Work out the finished part from the listing and answer in its coordinate system (mm). A direction names the side the tool comes from. Give positions to 0.01 mm unless a question says otherwise; leave off trailing zeros. Loops run counter-clockwise (first coordinate to the right, second up) from the corner with the lowest first, then second, coordinate; pieces in that order, holes last. Notation, with made-up numbers: (85.5, -26.5) - (109.5, -26.5) arc R20 ccw to (109.5, -9.5) - close; hole circle Ø1 at (1.25, 71.25). An arc over 180 degrees is marked (long way). One line per question, with ' | ' between items.
from build123d import *

# Parameters (mm, degrees)
SKETCH_1_R                                     = 31
FOOT_125X100_R10_T8_OPEN_D62_DEPTH             = 8
SKETCH_2_R                                     = 3.3
M6_GRID25_100X75_DEPTH                         = 8
SKETCH_3_R                                     = 34
SKETCH_3_R_2                                   = 31
HOLLOW_COLUMN_OD68_ID62_TOZ134_DEPTH           = 126
SKETCH_5_R                                     = 34
SKETCH_5_R_2                                   = 30.6
BOTTOM_CAP_WRAP_OD68_ID61P2_H6_DEPTH           = 6
STRAIGHT_TRIANGULAR_RIB_T4_NO_FILLETS_X_DEPTH  = 4
STRAIGHT_TRIANGULAR_RIB_T4_NO_FILLETS_Y_DEPTH  = 4
SKETCH_8_R                                     = 1.7
STATOR_4XM3_PCD25_THROUGH_WEB_DEPTH            = 6
SKETCH_9_R                                     = 3.3
UNDERSIDE_BOLT_AND_DRIVER_WELLS_D6P6_DEPTH     = 24
INNER_WALL_WIRE_GROOVE_W14_R2_DEPTH40_NO_DEPTH = 40
BOTTOM_REAR_OFFSET_WIRE_EXIT_14X10_45DEG_DEPTH = 25


with BuildPart() as part:
    # 草图1 → Foot_125x100_R10_T8_open_D62 (new body)
    with BuildSketch(Plane.XY):
        with BuildLine():
            Line((-52.5, -50), (52.5, -50))
            ThreePointArc((52.5, -50), (59.571067812, -47.071067812), (62.5, -40))
            Line((62.5, -40), (62.5, 40))
            ThreePointArc((62.5, 40), (59.571067812, 47.071067812), (52.5, 50))
            Line((52.5, 50), (-52.5, 50))
            ThreePointArc((-52.5, 50), (-59.571067812, 47.071067812), (-62.5, 40))
            Line((-62.5, 40), (-62.5, -40))
            ThreePointArc((-62.5, -40), (-59.571067812, -47.071067812), (-52.5, -50))
        make_face()
        Circle(SKETCH_1_R, mode=Mode.SUBTRACT)
    extrude(amount=FOOT_125X100_R10_T8_OPEN_D62_DEPTH)

    # 草图2 → M6_grid25_100x75 (cut)
    with BuildSketch(Plane.XY.offset(8)):
        with Locations((-50, -37.5)):
            Circle(SKETCH_2_R)
        with Locations((-50, 37.5)):
            Circle(SKETCH_2_R)
        with Locations((50, -37.5)):
            Circle(SKETCH_2_R)
        with Locations((50, 37.5)):
            Circle(SKETCH_2_R)
    extrude(amount=-M6_GRID25_100X75_DEPTH, mode=Mode.SUBTRACT)

    # 草图3 → Hollow_column_OD68_ID62_toZ134 (add)
    with BuildSketch(Plane.XY.offset(8)):
        Circle(SKETCH_3_R)
        Circle(SKETCH_3_R_2, mode=Mode.SUBTRACT)
    extrude(amount=HOLLOW_COLUMN_OD68_ID62_TOZ134_DEPTH)

    # 草图4 → Integral_motor_seat_45deg_internal_closure (revolve)
    with BuildSketch(Plane(origin=(0, 0, 0), x_dir=(1, 0, 0), z_dir=(0, 1, 0)), mode=Mode.PRIVATE) as integral_motor_seat_45deg_internal_closu_sk:
        Polygon((7, -131), (31, -107), (34, -107), (34, -134), (7, -134), align=None)
    revolve(integral_motor_seat_45deg_internal_closu_sk.sketch.rotate(Axis((0, 0, 0), (0, 0, 1)), 180), axis=Axis((0, 0, 0), (0, 0, 1)))

    # 草图5 → Bottom_cap_wrap_OD68_ID61p2_H6 (add)
    with BuildSketch(Plane.XY.offset(134)):
        Circle(SKETCH_5_R)
        Circle(SKETCH_5_R_2, mode=Mode.SUBTRACT)
    extrude(amount=BOTTOM_CAP_WRAP_OD68_ID61P2_H6_DEPTH)

    # 草图6 → Straight_triangular_rib_T4_no_fillets_x (add)
    with BuildSketch(Plane(origin=(-2, 0, 0), x_dir=(0, 0, -1), z_dir=(1, 0, 0))):
        Polygon((-8, -32), (-8, -46), (-22, -32), align=None)
        Polygon((-8, 32), (-8, 46), (-22, 32), align=None)
    extrude(amount=STRAIGHT_TRIANGULAR_RIB_T4_NO_FILLETS_X_DEPTH)

    # 草图7 → Straight_triangular_rib_T4_no_fillets_y (add)
    with BuildSketch(Plane(origin=(0, -2, 0), x_dir=(1, 0, 0), z_dir=(0, 1, 0))):
        Polygon((-32, -8), (-56, -8), (-32, -32), align=None)
        Polygon((32, -8), (56, -8), (32, -32), align=None)
    extrude(amount=STRAIGHT_TRIANGULAR_RIB_T4_NO_FILLETS_Y_DEPTH)

    # 草图8 → Stator_4xM3_PCD25_through_web (cut)
    with BuildSketch(Plane.XY.offset(134)):
        with Locations((12.5, 0)):
            Circle(SKETCH_8_R)
        with Locations((0, 12.5)):
            Circle(SKETCH_8_R)
        with Locations((-12.5, 0)):
            Circle(SKETCH_8_R)
        with Locations((0, -12.5)):
            Circle(SKETCH_8_R)
    extrude(amount=-STATOR_4XM3_PCD25_THROUGH_WEB_DEPTH, mode=Mode.SUBTRACT)

    # 草图9 → Underside_bolt_and_driver_wells_D6p6 (cut)
    with BuildSketch(Plane.XY.offset(128)):
        with Locations((12.5, 0)):
            Circle(SKETCH_9_R)
        with Locations((0, 12.5)):
            Circle(SKETCH_9_R)
        with Locations((-12.5, 0)):
            Circle(SKETCH_9_R)
        with Locations((0, -12.5)):
            Circle(SKETCH_9_R)
    extrude(amount=-UNDERSIDE_BOLT_AND_DRIVER_WELLS_D6P6_DEPTH, mode=Mode.SUBTRACT)

    # 草图10 → Inner_wall_wire_groove_W14_R2_depth40_no_external_bulge (cut)
    with BuildSketch(Plane.XY.offset(134)):
        with BuildLine():
            Line((-5, 19.5), (5, 19.5))
            ThreePointArc((5, 19.5), (6.414213562, 20.085786438), (7, 21.5))
            Line((7, 21.5), (7, 29.5))
            ThreePointArc((7, 29.5), (6.414213562, 30.914213562), (5, 31.5))
            Line((5, 31.5), (-5, 31.5))
            ThreePointArc((-5, 31.5), (-6.414213562, 30.914213562), (-7, 29.5))
            Line((-7, 29.5), (-7, 21.5))
            ThreePointArc((-7, 21.5), (-6.414213562, 20.085786438), (-5, 19.5))
        make_face()
    extrude(amount=-INNER_WALL_WIRE_GROOVE_W14_R2_DEPTH40_NO_DEPTH, mode=Mode.SUBTRACT)

    # 草图11 → Bottom_rear_offset_wire_exit_14x10_45deg_roof (cut)
    with BuildSketch(Plane(origin=(0, 40, 0), x_dir=(1, 0, 0), z_dir=(0, 1, 0))):
        Polygon((9, -8), (23, -8), (23, -18), (16, -25), (9, -18), align=None)
    extrude(amount=-BOTTOM_REAR_OFFSET_WIRE_EXIT_14X10_45DEG_DEPTH, mode=Mode.SUBTRACT)


solid = part.part
1. Find section D-D on z = 39. Write down the section's boundary in (x, y).
Evaluation:
outline: circle Ø68 at (0, 0); hole circle Ø62 at (0, 0)
2. Consider L1, parallel to Y at x = 0, z = 135; L2, parallel to Y at x = 0, z = 126; L3, parallel to Y at x = -9.5, z = 125. Determine where each line is inside the solid, lowest interval first.
Evaluation:
L1: -34 to -30.6, 30.6 to 34 | L2: -34 to -15.8, 15.8 to 19.5, 31.5 to 34 | L3: -32.65 to -8.87, 8.87 to 32.65
3. Which of the six approach directions +Z, -Z, +X, -X, +Y, -Y give full straight-line access (tool end or side, diameter ignored) to faces 4 (the flat face through (40, 2, 14)), 5 (the flat face through (2, -39, 13)), 6 (the flat face through (13, 30, 22)), 7 (the cylindrical face through (-6.633, -29.872, 136.958)), 8 (the flat face through (-14.2, 0.8, 128))?
Evaluation:
face 4: +Z, +X, +Y | face 5: +Z, +X, -Y | face 6: +Y | face 7: +Z | face 8: -Z
4. Find section B-B on y = 37.5. Write down the section's boundary in (x, z), then the cut area to 3 significant figures.
Evaluation:
outline: (-62.5, 0) - (-53.3, 0) - (-53.3, 8) - (-62.5, 8) - close; (-46.7, 0) - (46.7, 0) - (46.7, 8) - (2, 8) - (2, 16.5) - (-2, 16.5) - (-2, 8) - (-46.7, 8) - close; (53.3, 0) - (62.5, 0) - (62.5, 8) - (53.3, 8) - close | area: 928 mm2
5. Find section C-C on z = 103. Write down the section's boundary in (x, y), then the cut area to 3 significant figures.
Evaluation:
outline: circle Ø68 at (0, 0); hole (-6.86, 30.23) arc R31 ccw (long way) to (6.86, 30.23) arc R2 ccw to (5, 31.5) - (-5, 31.5) arc R2 ccw to start | area: 604 mm2
6. Find section A-A on x = 50. Write down the section's boundary in (y, z), then the cut area to 3 significant figures.
Evaluation:
outline: (-50, 0) - (-40.8, 0) - (-40.8, 8) - (-50, 8) - close; (-34.2, 0) - (34.2, 0) - (34.2, 8) - (2, 8) - (2, 14) - (-2, 14) - (-2, 8) - (-34.2, 8) - close; (40.8, 0) - (50, 0) - (50, 8) - (40.8, 8) - close | area: 718 mm2
7. Flat-ended cylindrical pins translate along their axes: pin 1 (4 mm diameter, centred on x = 12.5, y = 0, fed in from -Z); pin 2 (5 mm diameter, centred on x = 14, y = 0.5, fed in from -Z); pin 3 (11 mm diameter, centred on x = 2, z = 128, fed in from +Y); pin 4 (2 mm diameter, centred on x = -12.5, y = 0, fed in from -Z). Find the tip coordinate at first contact, or state that the pin passes through.
Evaluation:
pin 1: z = 128 | pin 2: z = 121.49 | pin 3: y = 34 | pin 4: through
8. Determine the mould class of faces 1 (the flat face through (-40, 2, 14)), 2 (the flat face through (-2, -13, 128)), 3 (the flat face through (-28, 13, 140)) for opening direction Y: +Y half, -Y half, draft (parallel to the pull), parting line (faces both ways), or undercut.
Evaluation:
face 1: +Y half | face 2: undercut | face 3: draft
